from build123d import *

# Parameters (mm, degrees)
SKETCH1_R           = 1.765617114
BOSS_EXTRUDE1_DEPTH = 300
SKETCH2_R           = 1.765617114
BOSS_EXTRUDE2_DEPTH = 300
SKETCH3_R           = 1.765617114
BOSS_EXTRUDE3_DEPTH = 300


with BuildPart() as part:
    # Sketch1 → Boss-Extrude1 (new body)
    with BuildSketch(Plane.XY):
        Circle(SKETCH1_R)
    extrude(amount=BOSS_EXTRUDE1_DEPTH)

    # Sketch2 → Boss-Extrude2 (add)
    with BuildSketch(Plane(origin=(0, 0, 0), x_dir=(0, 0, -1), z_dir=(1, 0, 0))):
        with Locations(Location((0, 0, 0), (0, 0, 90))):
            Circle(SKETCH2_R)
    extrude(amount=BOSS_EXTRUDE2_DEPTH)

    # Sketch3 → Boss-Extrude3 (add)
    with BuildSketch(Plane(origin=(0, 0, 0), x_dir=(1, 0, 0), z_dir=(0, 1, 0))):
        with Locations(Location((0, 0, 0), (0, 0, 90))):
            Circle(SKETCH3_R)
    extrude(amount=BOSS_EXTRUDE3_DEPTH)


solid = part.part
The listing builds one solid part. Answer for the finished solid, in the listing's coordinates (mm). Round coordinates to 2 decimals unless told otherwise and drop trailing zeros. Order: outer loops, then holes, each group sorted by start corner. A loop starts at its lowest first (then second) coordinate and runs counter-clockwise, first axis right, second up. Notation, with made-up numbers: M 32.5,-9.75 L 49.5,-9.75 A16 ccw 49.5,20.25 Z; hole C -30,-20.5 d11. An arc over 180 degrees is marked long. Answer in a Markdown table with one row per item. Add a question column.
1) Flat-ended cylindrical pins translate along their axes: pin 1 Ø0.9 at (x, z) = (-1, -1) entering from -Y; pin 2 Ø0.9 at (y, z) = (-1, -0.5) entering from -X; pin 3 Ø1.4 at (x, y) = (-1, -1) entering from -Z. Find the tip coordinate at first contact, or state that the pin passes through.
2) The part is cut by section A-A on z = 241. Determine the outline of the cut face in (x, y).
Findings below:
| question | item | result |
|---|---|---|
| 1 | pin 1 | stops at y = 0 |
| 1 | pin 2 | stops at x = 0 |
| 1 | pin 3 | stops at z = 0 |
| 2 | outline | C 0,0 d3.53 |
